For this review, take the finished solid that the model builds, in its own axes (mm). A direction names the side the tool comes from. Coordinates: 2 decimals unless noted, no trailing zeros. Loops run counter-clockwise (first coordinate to the right, second up) from the corner with the lowest first, then second, coordinate; pieces in that order, holes last.
1. Take a section at A-A, the plane y = -35. State the section outline as (x, z) points, then the cut area to 3 significant figures.
2. To check wall thickness, follow probe 1 along Y at (x, z) = (15, -9); probe 2 along Z at (x, y) = (-12.75, -52.5) (3 decimals); probe 3 along Y at (x, z) = (0, 1.35). State the ranges of each line that lie inside material, in increasing order.
3. Mouldability with a two-part tool opening along X and no side actions: class faces 5 (the face through (13.641, -28.797, -12.551)), 6 (the face through (-12, -44, -26.7)), 7 (the face through (-10.098, -8.387, 0.986)), 8 (the face through (-19.36, 0.9, 1.01)) as pulls with the +X half, pulls with the -X half, needs draft (parallel to the pull), parting line crosses it, or undercut.
4. Take a section at B-B, the plane x = 0. State the section outline as (y, z) points, then the cut area to 3 significant figures.
5. Take a section at D-D, the plane y = -1. State the section outline as (x, z) points, then the cut area to 3 significant figures.
6. Take a section at C-C, the plane z = -1. State the section outline as (x, y) points, then the cut area to 3 significant figures.
7. Machinability: for faces 1 (the face through (0, -30, -12)), 2 (the face through (0, 8, 0)), 3 (the face through (-13.641, -28.797, -12.149)), 4 (the face through (18, -30, -13)), which of the approach directions +Z, -Z, +X, -X, +Y, -Y give a long, thin tool a straight path to every point of the face, cutting with its end or side? Answer none if there is none.
8. Clearance check with flat-ended pins moving along their axes: P1, Ø8, axis at x = -18.5, z = -25, coming from the +Y side; P2, Ø4, axis at x = 15, y = -32, coming from the -Z side; P3, Ø12.5, axis at y = -40, z = -12.35, coming from the -X side; P4, Ø3.5, axis at x = 9.9, y = -9.9, coming from the +Z side. State where each tip first meets the part, or that it passes through.
```python
from build123d import *

# Parameters (mm, degrees)
SKETCH2_R               = 1.525
SKETCH2_R_2             = 7.5
BOSS_EXTRUDE3_DEPTH     = 2
BOSS_EXTRUDE4_START     = -40
BOSS_EXTRUDE4_DEPTH     = 42
BOSS_EXTRUDE6_START     = -30
SKETCH7_W               = 37.7
SKETCH7_H               = 28.7
SKETCH7_R               = 9.4
BOSS_EXTRUDE6_DEPTH     = 30
BOSS_EXTRUDE7_START     = -26.7
BOSS_EXTRUDE7_DEPTH     = 26.7
CUT_EXTRUDE1_DEPTH      = 76.921423195
CUT_EXTRUDE1_DEPTH_BACK = 76.921423195
SKETCH6_R               = 3.975
RIB3_START              = -5
RIB3_DEPTH              = 10
FILLET2_R               = 4


# Read off the part's stored shape, not the designer's step: Rib3
with BuildPart() as part:
    # Sketch2 → Boss-Extrude3 (new body)
    with BuildSketch(Plane.XY):
        with BuildLine():
            Line((12.5, -30), (12.5, -13.297086147))
            ThreePointArc((12.5, -13.297086147), (0, 18.25), (-12.5, -13.297086147))
            Line((-12.5, -13.297086147), (-12.5, -30))
            Line((-12.5, -30), (12.5, -30))
        make_face()
        with Locations((9.899494937, -9.899494937)):
            Circle(SKETCH2_R, mode=Mode.SUBTRACT)
        with Locations((-9.899494937, -9.899494937)):
            Circle(SKETCH2_R, mode=Mode.SUBTRACT)
        with Locations((-9.899494937, 9.899494937)):
            Circle(SKETCH2_R, mode=Mode.SUBTRACT)
        with Locations((9.899494937, 9.899494937)):
            Circle(SKETCH2_R, mode=Mode.SUBTRACT)
        Circle(SKETCH2_R_2, mode=Mode.SUBTRACT)
    extrude(amount=BOSS_EXTRUDE3_DEPTH)

    # Sketch3 → Boss-Extrude4 (add)
    with BuildSketch(Plane.XY.offset(BOSS_EXTRUDE4_START)):
        with BuildLine():
            Line((23.75, 0), (18.25, 0))
            ThreePointArc((18.25, 0), (0, -18.25), (-18.25, 0))
            Line((-18.25, 0), (-23.75, 0))
            ThreePointArc((-23.75, 0), (0, -23.75), (23.75, 0))
        make_face()
    extrude(amount=BOSS_EXTRUDE4_DEPTH)

    # Sketch7 → Boss-Extrude6 (add)
    with BuildSketch(Plane(origin=(0, 0, 0), x_dir=(1, 0, 0), z_dir=(0, 1, 0)).offset(BOSS_EXTRUDE6_START)):
        with Locations((0, 12.35)):
            Rectangle(SKETCH7_W, SKETCH7_H)
        with Locations(Location((0, 12.35, 0), (0, 0, 180))):
            Circle(SKETCH7_R, mode=Mode.SUBTRACT)
    extrude(amount=-BOSS_EXTRUDE6_DEPTH)

    # Sketch2<8> → Boss-Extrude7 (add)
    with BuildSketch(Plane.XY.offset(BOSS_EXTRUDE7_START)):
        with BuildLine():
            Line((12.5, -30), (12.5, -13.297086147))
            ThreePointArc((12.5, -13.297086147), (0, -18.25), (-12.5, -13.297086147))
            Line((-12.5, -13.297086147), (-12.5, -30))
            Line((-12.5, -30), (12.5, -30))
        make_face()
    extrude(amount=BOSS_EXTRUDE7_DEPTH)

    # Sketch6 → Cut-Extrude1 (cut, two sides: drawn at the far end of the back side and taken through both)
    with BuildSketch(Plane(origin=(0, 0, 0), x_dir=(0, 0, -1), z_dir=(1, 0, 0)).offset(-CUT_EXTRUDE1_DEPTH_BACK)):
        with Locations((12.35, -40)):
            Circle(SKETCH6_R)
        with Locations((12.35, -52.5)):
            Circle(SKETCH6_R)
    extrude(amount=CUT_EXTRUDE1_DEPTH + CUT_EXTRUDE1_DEPTH_BACK, mode=Mode.SUBTRACT)

    # Rib3 outline → Rib3 (add)
    with BuildSketch(Plane(origin=(0, -60, 0), x_dir=(0, -1, 0), z_dir=(-1, 0, 0)).offset(RIB3_START)):
        Polygon((-38, -40), (-31.25, -40), (0, -26.7), (-38, -26.7), align=None)
    extrude(amount=RIB3_DEPTH)

    # Fillet2
    fillet2_edges = [part.edges().sort_by_distance(p)[0] for p in [
        (12.5, -30, -12.35),
        (-12.5, -30, -12.35),
        (-18.25, 0, 1),
        (12.5, -20.194368027, -12.35),
        (18.25, 0, 1),
        (-12.5, -20.194368027, -12.35),
    ]]
    fillet(fillet2_edges, radius=FILLET2_R)


solid = part.part
```
Results list:
1. outline: (-18.85, -26.7) - (-5, -26.7) - (-5, -37.34) - (5, -37.34) - (5, -26.7) - (18.85, -26.7) - (18.85, 2) - (-18.85, 2) - close; hole circle Ø18.8 at (0, -12.35)
1. area: 911 mm2
2. probe 1: y = -60 to -54.64, -50.36 to -42.14, -37.86 to -29.71, -18.41 to -10.4
2. probe 2: z = -26.7 to -16.325, -8.375 to 2
2. probe 3: y = -60 to -7.5, 7.5 to 18.25
3. face 5: pulls with the +X half
3. face 6: needs draft
3. face 7: undercut
3. face 8: pulls with the -X half
4. outline: (-60, -26.7) - (-28.75, -40) - (-18.25, -40) - (-18.25, 0) - (-7.5, 0) - (-7.5, 2) - (-60, 2) - (-60, -2.95) - (-30, -2.95) - (-30, -21.75) - (-60, -21.75) - close; (7.5, 0) - (18.25, 0) - (18.25, 2) - (7.5, 2) - close
4. area: 1,020 mm2
5. outline: (-23.73, -40) - (-18.22, -40) - (-18.22, 0) - (-7.43, 0) - (-7.43, 2) - (-23.73, 2) - close; (7.43, 0) - (18.22, 0) - (18.22, -40) - (23.73, -40) - (23.73, 2) - (7.43, 2) - close
5. area: 506 mm2
6. outline: (-23.75, 0) arc R23.75 ccw to (-14.12, -19.1) arc R4 cw to (-12.5, -22.31) - (-12.5, -26) arc R4 cw to (-16.5, -30) - (-18.85, -30) - (-18.85, -60) - (18.85, -60) - (18.85, -30) - (16.5, -30) arc R4 cw to (12.5, -26) - (12.5, -22.31) arc R4 cw to (14.12, -19.1) arc R23.75 ccw to (23.75, 0) - (18.25, 0) arc R18.25 cw to (-18.25, 0) - close
6. area: 1,690 mm2
7. face 1: -Y
7. face 2: -Z, +Y
7. face 3: +Z, -Z, -X
7. face 4: +Z, -Z, +X
8. P1: stops at y = 0
8. P2: stops at z = -26.7
8. P3: stops at x = -18.85
8. P4: stops at z = 2
